Design review of the part shown in the three views and the two pictorial views. Dimensions are in mm from the part's minimum x, y and z. A direction names the side the tool comes from. Give positions to 0.01 mm unless a question says otherwise; leave off trailing zeros. Order: outer loops, then holes, each group sorted by start corner. A loop starts at its lowest first (then second) coordinate and runs counter-clockwise, first axis right, second up. Notation, with made-up numbers: (70.5, 86.5) - (120.5, 86.5) arc R12 cw to (120.5, 92.5) - close; hole circle Ø9 at (-33, -5.5). An arc over 180 degrees is marked (long way). Put each result on its own line as item: value.
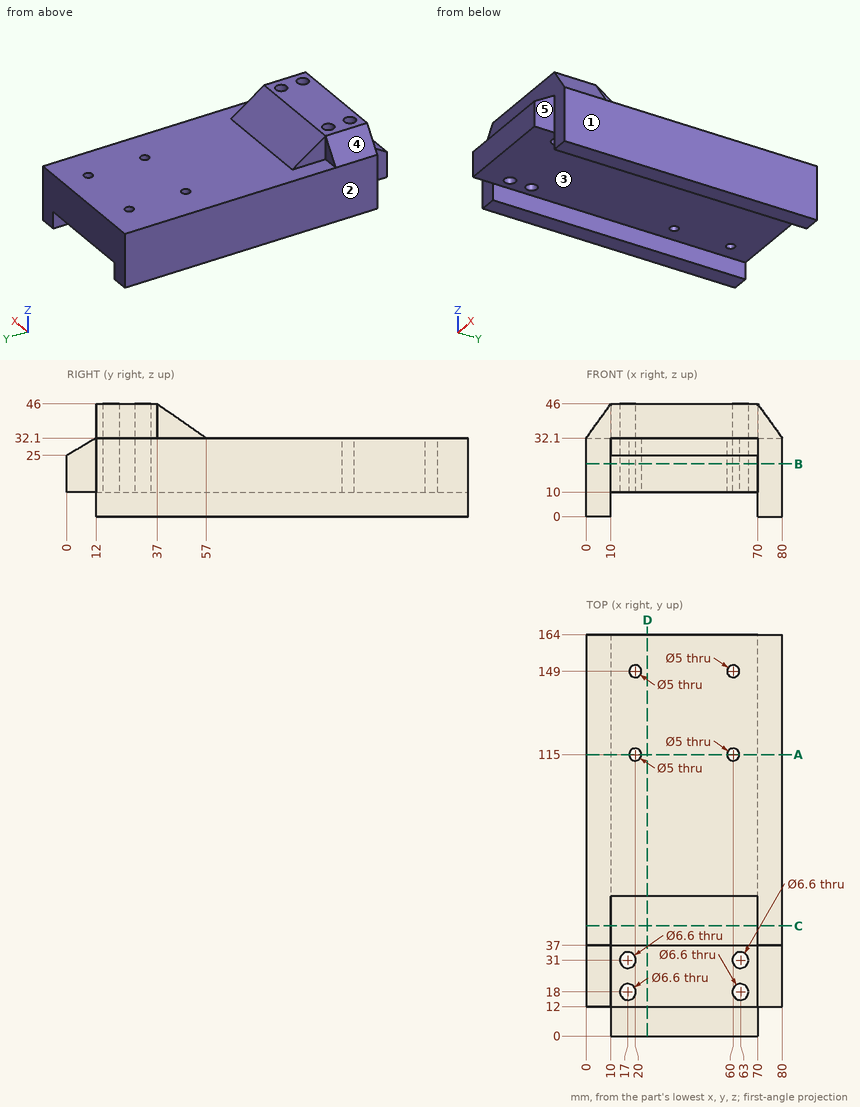
(1) Take a section at B-B, the plane z = 21.5. Count the separate pieces of the cut face and the enclosed holes in it, then the cut area to 3 significant figures.
The answers:
separate pieces: 1
enclosed holes: 8
area: 12,700 mm^2
(2) Clearance check with flat-ended pins moving along their axes: pin 1 Ø6 at (x, y) = (20, 115) entering from +Z; pin 2 Ø5.5 at (x, y) = (17, 18) entering from +Z; pin 3 Ø8 at (x, z) = (29, 31) entering from -Y; pin 4 Ø6.5 at (x, y) = (20, 149) entering from -Z. State where each tip first meets the part, or that it passes through.
The answers:
pin 1: z = 32.1
pin 2: through
pin 3: y = 3.38
pin 4: z = 10
(3) For the marked faces 4 and 5, list the 3-axis set-ups (+Z, -Z, +X, -X, +Y, -Y) from which the entire face can be reached by the end or side of a thin tool; tool diameter is ignored.
The answers:
face 4: +Z, -X, +Y, -Y
face 5: +Z, -Z, +X, -Y
(4) Take a section at A-A, the plane y = 115. Write out the cut boundary in (x, z).
The answers:
outline: (0, 0) - (10, 0) - (10, 10) - (17.5, 10) - (17.5, 32.1) - (0, 32.1) - close; (22.5, 10) - (57.5, 10) - (57.5, 32.1) - (22.5, 32.1) - close; (62.5, 10) - (70, 10) - (70, 0) - (80, 0) - (80, 32.1) - (62.5, 32.1) - close
(5) Take a section at D-D, the plane x = 25. Write out the cut boundary in (y, z).
The answers:
outline: (0, 10) - (164, 10) - (164, 32.1) - (57, 32.1) - (37, 46) - (12, 46) - (12, 32.1) - (0, 25) - close
(6) The part is to be moulded in two halves that separate along X. For the marked faces 1, 2 and 3, say which applies: pulls with the +X half, pulls with the -X half, needs draft (parallel to the pull), parting line crosses it, or undercut.
The answers:
face 1: pulls with the +X half
face 2: pulls with the -X half
face 3: undercut
(7) Take a section at C-C, the plane y = 45. Write out the cut boundary in (x, z), then the cut area to 3 significant figures.
The answers:
outline: (0, 0) - (10, 0) - (10, 10) - (70, 10) - (70, 0) - (80, 0) - (80, 32.1) - (70, 32.1) - (70, 40.44) - (10, 40.44) - (10, 32.1) - (0, 32.1) - close
area: 2,470 mm^2
(8) Wall thickness on L1, parallel to Y at x = 17, z = 18; L2, parallel to X at y = 149, z = 27; L3, parallel to Y at x = 20, z = 16.75: over which ranges is each line inside the solid? List them lowest first.
The answers:
L1: 0 to 14.7, 21.3 to 27.7, 34.3 to 164
L2: 0 to 17.5, 22.5 to 57.5, 62.5 to 80
L3: 0 to 16.63, 19.37 to 29.63, 32.37 to 112.5, 117.5 to 146.5, 151.5 to 164
